from build123d import *

# Parameters (mm, degrees)
SKETCH002_R  = 8.5
PAD001_DEPTH = 15
SKETCH003_R  = 7
POCKET_DEPTH = 28
CHAMFER_SIZE = 0.5


with BuildPart() as part:
    # Sketch002 (on Face1 of ReferenceFillet) → Pad001 (new body)
    with BuildSketch(Plane(origin=(0, 0, 0), x_dir=(1, 0, 0), z_dir=(0, 0, -1))):
        with Locations((-24.532044, 0)):
            Circle(SKETCH002_R)
    extrude(amount=PAD001_DEPTH)

    # Sketch003 (on Face3 of Pad001) → Pocket (cut)
    with BuildSketch(Plane(origin=(0, 0, -15), x_dir=(1, 0, 0), z_dir=(0, 0, -1))):
        with Locations((-24.47134, 0)):
            Circle(SKETCH003_R)
    extrude(amount=-POCKET_DEPTH, mode=Mode.SUBTRACT)

    # Chamfer
    chamfer_edges = [part.edges().sort_by_distance(p)[0] for p in [
        (-31.47134, 0, -15),
    ]]
    chamfer(chamfer_edges, length=CHAMFER_SIZE)


solid = part.part
Work out the finished part from the listing and answer in its coordinate system (mm). Give positions to 0.01 mm unless a question says otherwise; leave off trailing zeros. Write each loop counter-clockwise with the first axis right and the second up, starting at its lowest first coordinate (ties: lowest second). Pieces come first, ordered by that corner, then holes. Notation, with made-up numbers: (-36.75, -24.75) - (22.25, -24.75) arc R24 cw to (22.25, 2.25) - close; hole circle Ø3 at (3, 0.25). An arc over 180 degrees is marked (long way). One line per item, written item: value. Start each with the question number.
1. For a pull along Y with two mould halves and no side action, classify faces 1 (the cylindrical face through (-16.425, -2.553, -7.395)), 2 (the flat face through (-30, -6, -15)), 3 (the cylindrical face through (-18.005, 2.681, -7.352)) as +Y half, -Y half, draft (parallel to the pull), parting line (faces both ways), or undercut.
2. Given pin 1 (1.5 mm diameter, centred on y = -6.5, z = -2, fed in from +X); pin 2 (2 mm diameter, centred on x = -18.5, z = -7.5, fed in from +Y); pin 3 (2 mm diameter, centred on y = -6.5, z = -8, fed in from +X), each flat-ended and moving along its own axis, determine where each tip first touches the part or whether it passes through.
3. Find section B-B (z = -3.25). Write down the section's boundary in (x, y).
4. Find section A-A (y = 0). Write down the section's boundary in (x, z), then the cut area to 4 significant figures.
5. Consider probe 1 along X at (y, z) = (0, -3); probe 2 along Y at (x, z) = (-24.5, -7.5); probe 3 along Y at (x, z) = (-29.75, -11). Determine where each line is inside the solid, lowest interval first.
Geometry results:
1. face 1: parting line
1. face 2: draft
1. face 3: undercut
2. pin 1: x = -18.27
2. pin 2: y = 6.85
2. pin 3: x = -18.05
3. outline: circle Ø17 at (-24.53, 0); hole circle Ø14 at (-24.47, 0)
4. outline: (-33.03, -15) - (-31.97, -15) - (-31.47, -14.5) - (-31.47, 0) - (-33.03, 0) - close; (-17.47, -14.5) - (-16.97, -15) - (-16.03, -15) - (-16.03, 0) - (-17.47, 0) - close
4. area: 44.75 mm2
5. probe 1: -33.03 to -31.47, -17.47 to -16.03
5. probe 2: -8.5 to -7, 7 to 8.5
5. probe 3: -6.71 to -4.6, 4.6 to 6.71
